Design review of the part shown in the three views and the two pictorial views. Dimensions are in mm from the part's minimum x, y and z. Round coordinates to 2 decimals unless told otherwise and drop trailing zeros. Order: outer loops, then holes, each group sorted by start corner. A loop starts at its lowest first (then second) coordinate and runs counter-clockwise, first axis right, second up. Notation, with made-up numbers: (24, -29.5) - (44, -29.5) arc R31 cw to (44, 6.5) - close; hole circle Ø2 at (16.5, 50). An arc over 180 degrees is marked (long way). One line per item, written item: value.
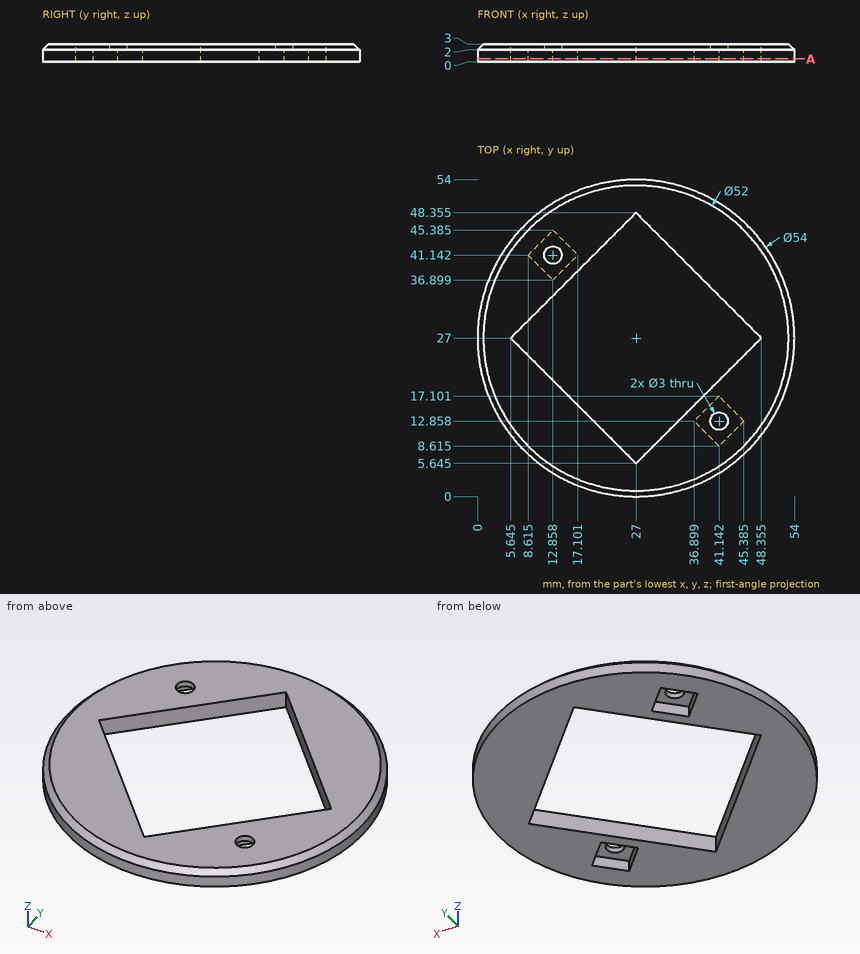
Item 1: For P1, Ø1.5, axis at y = 26, z = 2.5, coming from the -X side; P2, Ø9.5, axis at x = 39, y = 13, coming from the -Z side; P3, Ø1.5, axis at x = 37.5, z = 0.5, coming from the +Y side; P4, Ø3.5, axis at x = 12.86, y = 41.14, coming from the -Z side, all flat-tipped, find the tip position at first contact; note any pin that passes through.
Returned:
P1: x = 0
P2: z = 0
P3: y = 52.18
P4: z = 2
Item 2: Wall thickness on line 1 (X direction, y = 45, z = 1.85) (1 decimal); line 2 (Y direction, x = 38, z = 1.6) (1 decimal); line 3 (X direction, y = 13, z = 0.65) (1 decimal): over which ranges is each line inside the solid? List them lowest first.
Returned:
line 1: 6.9 to 12.5, 13.2 to 23.6, 30.4 to 47.1
line 2: 2.3 to 11.8, 14 to 16.6, 37.4 to 51.7
line 3: 3.9 to 19.6, 34.4 to 37, 45.2 to 50.1
Item 3: Take a section at A-A (z = 0.45). Write out the cut boundary in (x, y) (1 decimal).
Returned:
outline: circle Ø54 at (27, 27); hole (5.6, 27) - (27, 5.6) - (48.4, 27) - (27, 48.4) - close; hole (8.6, 41.1) - (12.9, 36.9) - (17.1, 41.1) - (12.9, 45.4) - close; hole (36.9, 12.9) - (41.1, 8.6) - (45.4, 12.9) - (41.1, 17.1) - close
